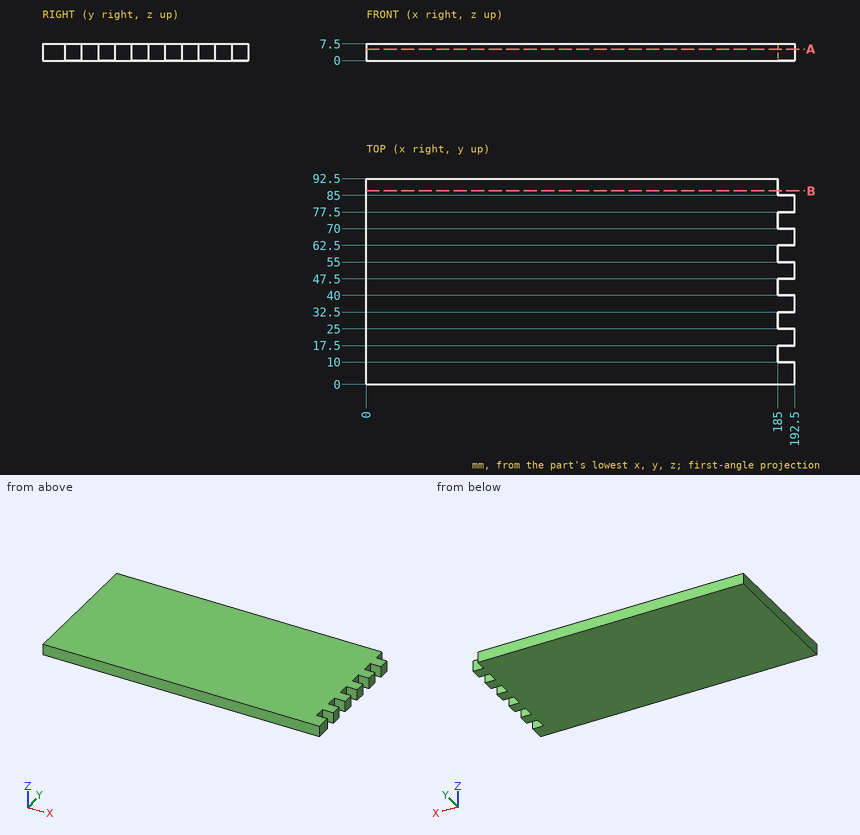
For this review, use the dimensioned drawing (mm, ordinates from the lowest corner) and the shaded views. Round coordinates to 2 decimals unless told otherwise and drop trailing zeros. Order: outer loops, then holes, each group sorted by start corner. A loop starts at its lowest first (then second) coordinate and runs counter-clockwise, first axis right, second up. Notation, with made-up numbers: M 40.25,-33 L 88.25,-33 A27 ccw 88.25,5 Z; hole C 40,16 d10. An arc over 180 degrees is marked long. Use a Markdown table: item, result. Add a question column.
Item 1: Add section B-B, the plane y = 87. Give the boundary of the cut face in (x, z).
Item 2: Add section A-A, the plane z = 5.25. Give the boundary of the cut face in (x, y), then the cut area to 3 significant figures.
Item 3: Insertion check: pin 1 (2 mm diameter, centred on x = 189.5, z = 3, fed in from +Y); pin 2 (1.5 mm diameter, centred on x = 108, y = 44, fed in from -Z); pin 3 (4 mm diameter, centred on y = 44.5, z = 2.5, fed in from +X). Each pin has a flat end and moves straight along its axis. Give the tip position at first contact, or say it passes through.
Item 4: To check wall thickness, follow line 1 along X through (y, z) = (27.5, 1.25). State the ranges of the line that lie inside material, in increasing order.
Geometry results:
| question | item | result |
|---|---|---|
| 1 | outline | M 0,0 L 185,0 L 185,7.5 L 0,7.5 Z |
| 2 | outline | M 0,0 L 192.5,0 L 192.5,10 L 185,10 L 185,17.5 L 192.5,17.5 L 192.5,25 L 185,25 L 185,32.5 L 192.5,32.5 L 192.5,40 L 185,40 L 185,47.5 L 192.5,47.5 L 192.5,55 L 185,55 L 185,62.5 L 192.5,62.5 L 192.5,70 L 185,70 L 185,77.5 L 192.5,77.5 L 192.5,85 L 185,85 L 185,92.5 L 0,92.5 Z |
| 2 | area | 17,500 mm² |
| 3 | pin 1 | stops at y = 85 |
| 3 | pin 2 | stops at z = 0 |
| 3 | pin 3 | stops at x = 185 |
| 4 | line 1 | x = 0 to 185 |
